Could you check a few things on this model? Use its own coordinates, in mm. Round coordinates to 2 decimals unless told otherwise and drop trailing zeros. Loops run counter-clockwise (first coordinate to the right, second up) from the corner with the lowest first, then second, coordinate; pieces in that order, holes last. Notation, with made-up numbers: M 72.25,-40 L 94.25,-40 A12 ccw 94.25,-30 Z; hole C 19.25,-38.5 d11. An arc over 180 degrees is marked long. One line per item, written item: value. Start each with the question number.
Q1. I'm going to push a flat-ended pin straight in: pin 1 Ø8 at (x, y) = (65.5, 17) entering from +Z. Where does the tip first touch, or does it pass through?
Q2. Please list where these lines run through material, in increasing order: line 1 along Z through (x, y) = (-119, 10.75); line 2 along Z through (x, y) = (80, 11); line 3 along X through (y, z) = (18.25, 113.5).
Q3. Imagine slicing it at A-A (y = 16.5). Please give me the cut outline in (x, z).
from build123d import *

# Parameters (mm, degrees)
BOSS_EXTRUDE1_DEPTH = 20
FILLET1_R           = 10


with BuildPart() as part:
    # Sketch1 → Boss-Extrude1 (new body)
    with BuildSketch(Plane(origin=(0, 0, 0), x_dir=(1, 0, 0), z_dir=(0, 1, 0))):
        with BuildLine():
            Line((-145, -200), (145, -200))
            ThreePointArc((145, -200), (166.213203436, -191.213203436), (175, -170))
            Line((175, -170), (175, 170))
            ThreePointArc((175, 170), (166.213203436, 191.213203436), (145, 200))
            Line((145, 200), (-145, 200))
            ThreePointArc((-145, 200), (-166.213203436, 191.213203436), (-175, 170))
            Line((-175, 170), (-175, -170))
            ThreePointArc((-175, -170), (-166.213203436, -191.213203436), (-145, -200))
        make_face()
    extrude(amount=BOSS_EXTRUDE1_DEPTH)

    # Fillet1
    fillet1_edges = [part.edges().sort_by_distance(p)[0] for p in [
        (166.213203436, 20, 191.213203436),
        (175, 20, 0),
        (166.213203436, 20, -191.213203436),
        (0, 20, -200),
        (-166.213203436, 20, -191.213203436),
        (-175, 20, 0),
        (-166.213203436, 20, 191.213203436),
        (0, 20, 200),
    ]]
    fillet(fillet1_edges, radius=FILLET1_R)


solid = part.part
Report:
1. pin 1: stops at z = 199.54
2. line 1: z = -199.97 to 199.97
2. line 2: z = -199.95 to 199.95
2. line 3: x = -170.65 to 170.65
3. outline: M -172.6,-170 A27.6 ccw -145,-197.6 L 145,-197.6 A27.6 ccw 172.6,-170 L 172.6,170 A27.6 ccw 145,197.6 L -145,197.6 A27.6 ccw -172.6,170 Z
